Verification items for the finished model (mm, model axes). Face numbers are marked on the shaded views. A direction names the side the tool comes from. Give positions to 0.01 mm unless a question says otherwise; leave off trailing zeros. Write each loop counter-clockwise with the first axis right and the second up, starting at its lowest first coordinate (ties: lowest second). Pieces come first, ordered by that corner, then holes. Notation, with made-up numbers: M 14.25,-27 L 42.25,-27 A26 cw 42.25,6 Z; hole C 50.25,35 d1. An arc over 180 degrees is marked long. Answer as a JSON object with one key per item and string values.
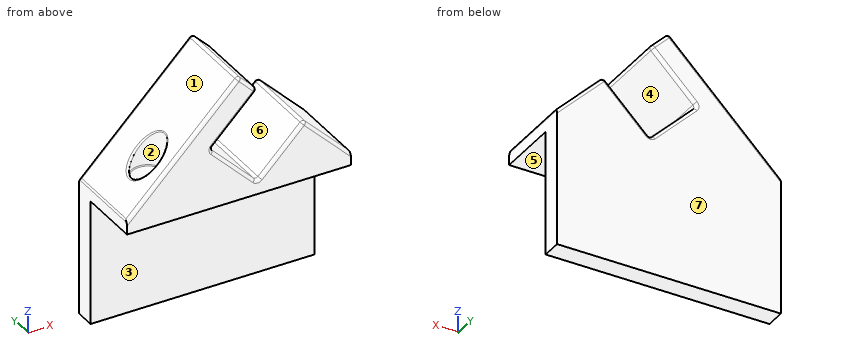
```python
from build123d import *

# Parameters (mm, degrees)
F1_DEPTH    = 25
F2_W        = 19.05
F2_H        = 38.1
F3_DEPTH    = 68.1660937064
F4_F1_R     = 1
F4_F2_R     = 1
F5_R        = 5
F5_R_2      = 1.5875
F6_DEPTH    = 37.6693332908
F7_DEPTH    = 10
F8_S5_R     = 5
F8_T6_DEPTH = 10
F9_R        = 0.5


# Not quite as in the source:
# - a fillet or chamfer that OpenCascade refuses, or shapes differently, is made with other operations: its cross-section is extruded or revolved along the edge and cut away or added


with BuildPart() as f1:
    # F0 (on Front) → F1 (new body)
    with BuildSketch(Plane.XZ):
        Polygon((-34.0825468532, 76.1825468532), (-68.1650937064, 42.1), (-68.1650937064, 0), (0, 0), (0, 42.1), (-14.2128463018, 56.3128463018), (-28.4256926037, 42.1), (-42.6385389055, 56.3128463018), (-28.4256926037, 70.5256926037), align=None)
    extrude(amount=F1_DEPTH)

    # F2 (on face) → F3 (cut, through all)
    with BuildSketch(Plane.YZ):
        with Locations((-15.475, 19.05)):
            Rectangle(F2_W, F2_H)
    extrude(amount=-F3_DEPTH, mode=Mode.SUBTRACT)

    # F4: fillet of radius 1 on 17 edges, made by hand

    # F4_f1
    f4_f1_edges = [f1.edges().sort_by_distance(p)[0] for p in [
        (-42.6385389055, -12.5, 56.3128463018),
        (-28.4256926037, -12.5, 42.1),
    ]]
    fillet(f4_f1_edges, radius=F4_F1_R)

    # F4_f2
    f4_f2_edges = [f1.edges().sort_by_distance(p)[0] for p in [
        (-28.4256926037, -12.5, 70.5256926037),
        (-35.178562364, 0, 63.7728228434),
        (-35.178562364, -25, 63.7728228434),
        (-14.2128463018, -12.5, 56.3128463018),
        (-20.9657160622, 0, 49.5599765415),
        (-20.9657160622, -25, 49.5599765415),
        (-34.0825468532, -12.5, 76.1825468532),
        (-68.1650937064, -12.5, 42.1),
        (-51.1238202798, 0, 59.1412734266),
        (-51.1238202798, -25, 59.1412734266),
        (0, -12.5, 42.1),
        (-7.1064231509, 0, 49.2064231509),
        (-7.1064231509, -25, 49.2064231509),
        (-31.2541197284, 0, 73.3541197284),
        (-31.2541197284, -25, 73.3541197284),
        (-28.4256926037, -25, 42.5142135624),
        (-28.4256926037, 0, 42.5142135624),
        (-42.2243253432, -25, 56.3128463018),
        (-42.2243253432, 0, 56.3128463018),
    ]]
    fillet(f4_f2_edges, radius=F4_F2_R)

    # F5 (on face) → F6 (cut, through all)
    with BuildSketch(Plane(origin=(0, 0, 38.1), x_dir=(1, 0, 0), z_dir=(0, 0, -1))):
        with Locations((-56.1650937064, 15.475)):
            Circle(F5_R)
        with Locations((-56.1650937064, 15.475)):
            Circle(F5_R_2, mode=Mode.SUBTRACT)
        with Locations((-56.1650937064, 15.475)):
            Circle(F5_R_2)
    extrude(amount=-F6_DEPTH, mode=Mode.SUBTRACT)

    # F5 (on face) → F7 (join)
    with BuildSketch(Plane(origin=(0, 0, 38.1), x_dir=(1, 0, 0), z_dir=(0, 0, -1))):
        with Locations((-56.1650937064, 15.475)):
            Circle(F5_R)
        with Locations((-56.1650937064, 15.475)):
            Circle(F5_R_2, mode=Mode.SUBTRACT)
    extrude(amount=-F7_DEPTH)

    # F8: chamfer of 4 on 1 edges, made by hand


with BuildPart() as f8_tool2:
    # F8_s3 → F8_t4 (revolve)
    with BuildSketch(Plane.XZ.offset(15.475)):
        Polygon((-54.5775937064, 44.1), (-50.5775937064, 48.1), (-54.5775937064, 48.1), align=None)
    revolve(axis=Axis((-56.1650937064, -15.475, 48.1), (0, 0, -1)))

    # F8_s5 → F8_t6 (intersect, symmetric)
    with BuildSketch(Plane.XY.offset(46.1)):
        with Locations((-56.1650937064, -15.475)):
            Circle(F8_S5_R)
    extrude(amount=F8_T6_DEPTH, both=True, mode=Mode.INTERSECT)


with BuildPart() as f1_1:
    add(f1.part)

    # F8_t1: cut F8_tool2
    add(f8_tool2.part, mode=Mode.SUBTRACT)

    # F9
    f9_edges = [f1_1.edges().sort_by_distance(p)[0] for p in [
        (-61.165093, -15.47181, 49.100001),
        (-51.165094, -15.475, 53.30625),
        (-61.165094, -15.475, 47.5125),
        (-57.752594, -15.475, 44.1),
    ]]
    fillet(f9_edges, radius=F9_R)


solid = f1_1.part
```
1) Go/stop test with flat-tipped pins: pin 1 (4 mm diameter, centred on x = -49, y = -6, fed in from +Z); pin 2 (4 mm diameter, centred on y = -18.5, z = 50.5, fed in from +X); pin 3 (4 mm diameter, centred on x = -56.17, y = -15.48, fed in from +Z). Record where each tip stops, or that it passes through.
Completed:
{"pin 1": "stops at z = 63.27", "pin 2": "stops at x = -6.4", "pin 3": "stops at z = 44.52"}
2) Access from +Z, -Z, +X, -X, +Y, -Y to the whole of each face (thin tool, end or side, straight path). Record for the marked faces 1, 2 and 3.
Completed:
{"face 1": "+Z, -X, +Y, -Y", "face 2": "+Z", "face 3": "-Z, +X, -X, -Y"}
3) Section check B-B on z = 25. Record the boundary of the cut face in (x, y).
Completed:
{"outline": "M -68.17,-5.95 L 0,-5.95 L 0,0 L -68.17,0 Z"}
4) Release check for a two-part mould opening along Z. For the marked faces 4, 5, 6 and 7 record: pulls with the +Z half, pulls with the -Z half, needs draft (parallel to the pull), parting line crosses it, or undercut.
Completed:
{"face 4": "undercut", "face 5": "pulls with the -Z half", "face 6": "pulls with the +Z half", "face 7": "needs draft"}
5) Section check A-A on y = -5. Record the boundary of the cut face in (x, z), and give its area (3 significant figures).
Completed:
{"outline": "M -68.17,0 L 0,0 L 0,41.69 A1 ccw -0.29,42.39 L -13.51,55.61 A1 ccw -14.92,55.61 L -27.72,42.81 A1 cw -29.13,42.81 L -41.93,55.61 A1 cw -41.93,57.02 L -29.13,69.82 A1 ccw -29.13,71.23 L -33.38,75.48 A1 ccw -34.79,75.48 L -67.87,42.39 A1 ccw -68.17,41.69 Z", "area": "3,630 mm2"}
6) Thickness scan on L1, parallel to Y at x = -7.5, z = 15; L2, parallel to X at y = -11.5, z = 53; L3, parallel to X at y = -11.5, z = 46. Record the ranges inside material, lowest first.
Completed:
{"L1": "y = -5.95 to 0", "L2": "x = -53.13 to -39.33, -17.53 to -10.9", "L3": "x = -64.27 to -32.33, -24.53 to -3.9"}
